```python
from build123d import *

# Parameters (mm, degrees)
BOSS_EXTRUDE1_DEPTH     = 50.8
SKETCH3_R               = 4.9022
CUT_EXTRUDE1_DEPTH      = 50.8
SKETCH4_R               = 1.4732
CUT_EXTRUDE2_DEPTH      = 50.8
FILLET1_R               = 2.54
SKETCH5_W               = 25.4
SKETCH5_H               = 31.75
CUT_EXTRUDE3_DEPTH      = 27.924
CUT_EXTRUDE3_DEPTH_BACK = 5.826


with BuildPart() as part:
    # Sketch2 → Boss-Extrude1 (new body)
    with BuildSketch(Plane(origin=(0, 0, 0), x_dir=(0, 0, -1), z_dir=(1, 0, 0))):
        Polygon((0, 0), (31.75, 0), (31.75, 31.75), (26.924, 31.75), (26.924, 4.826), (0, 4.826), align=None)
    extrude(amount=-BOSS_EXTRUDE1_DEPTH)

    # Sketch3 → Cut-Extrude1 (cut)
    with BuildSketch(Plane.XY.offset(-26.924)):
        with Locations((-38.1, 19.05)):
            Circle(SKETCH3_R)
        with Locations((-12.7, 19.05)):
            Circle(SKETCH3_R)
    extrude(amount=-CUT_EXTRUDE1_DEPTH, mode=Mode.SUBTRACT)

    # Sketch4 → Cut-Extrude2 (cut)
    with BuildSketch(Plane(origin=(0, 4.826, 0), x_dir=(1, 0, 0), z_dir=(0, 1, 0))):
        with Locations((-44.45, 12.7)):
            Circle(SKETCH4_R)
        with Locations((-31.75, 12.7)):
            Circle(SKETCH4_R)
    extrude(amount=-CUT_EXTRUDE2_DEPTH, mode=Mode.SUBTRACT)

    # Fillet1
    fillet1_edges = [part.edges().sort_by_distance(p)[0] for p in [
        (-25.4, 4.826, 0),
        (-25.4, 31.75, -26.924),
    ]]
    fillet(fillet1_edges, radius=FILLET1_R)

    # Sketch5 → Cut-Extrude3 (cut, two sides)
    with BuildSketch(Plane.XY.offset(-26.924)) as cut_extrude3_sk:
        with Locations((-12.7, 15.875)):
            Rectangle(SKETCH5_W, SKETCH5_H)
    extrude(amount=CUT_EXTRUDE3_DEPTH, mode=Mode.SUBTRACT)
    extrude(cut_extrude3_sk.sketch, amount=-CUT_EXTRUDE3_DEPTH_BACK, mode=Mode.SUBTRACT)


solid = part.part
```
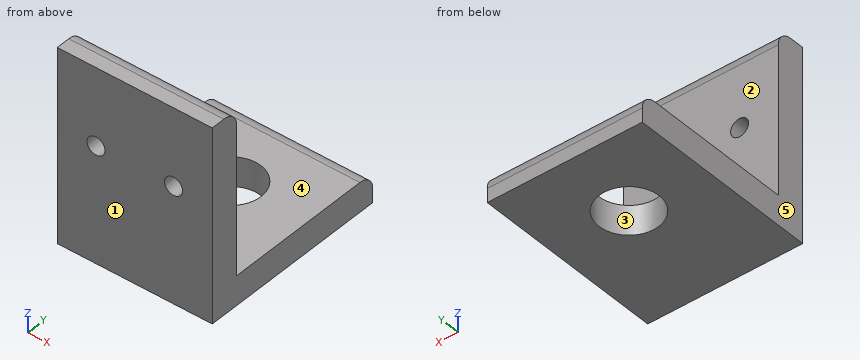
Input: part model. Units: mm. Frame: model coordinates. Face numbers are marked on the shaded views. A direction names the side the tool comes from. Round coordinates to 2 decimals unless told otherwise and drop trailing zeros. Order: outer loops, then holes, each group sorted by start corner. A loop starts at its lowest first (then second) coordinate and runs counter-clockwise, first axis right, second up. Notation, with made-up numbers: (83, 86.5) - (100, 86.5) arc R15 cw to (100, 101.5) - close; hole circle Ø5 at (26.25, 0.5). An arc over 180 degrees is marked (long way). Answer in a Markdown table with one row per item.
Item 1: Section query D-D (x = -48). Return the cut outline in (y, z), then the cut area to 3 significant figures.
Model answer:
| item | result |
|---|---|
| outline | (0, -31.75) - (31.75, -31.75) - (31.75, -29.46) arc R2.54 ccw to (29.21, -26.92) - (4.83, -26.92) - (4.83, -2.54) arc R2.54 ccw to (2.29, 0) - (0, 0) - close |
| area | 280 mm² |
Item 2: Line query: line 1 (X direction, y = 1.4, z = -12.7); line 2 (Z direction, x = -31.75, y = 1.15); line 3 (X direction, y = 1, z = -12). Output: solid intervals per line, ascending.
Model answer:
| item | result |
|---|---|
| line 1 | x = -50.8 to -45.92, -42.98 to -33.22, -30.28 to -25.4 |
| line 2 | z = -31.75 to -14.17, -11.23 to 0 |
| line 3 | x = -50.8 to -45.75, -43.15 to -33.05, -30.45 to -25.4 |
Item 3: Mould query, pull axis X, two halves, no side actions, for the marked faces 3, 4 and 5. Classes: released by +X, released by -X, zero draft, split by the parting line, or undercut.
Model answer:
| item | result |
|---|---|
| face 3 | undercut |
| face 4 | zero draft |
| face 5 | released by -X |
Item 4: Pin query (flat end, axial travel): pin 1 (10 mm diameter, centred on x = -36.5, z = -10, fed in from +Y); pin 2 (12 mm diameter, centred on x = -39.5, y = 22, fed in from +Z); pin 3 (1.8 mm diameter, centred on x = -44.45, z = -12.7, fed in from +Y). Return the tip coordinate at first contact, or that it passes through.
Model answer:
| item | result |
|---|---|
| pin 1 | stops at y = 4.83 |
| pin 2 | stops at z = -26.92 |
| pin 3 | passes through |
Item 5: Section query A-A (z = -12.7). Return the cut outline in (x, y), then the cut area to 3 significant figures.
Model answer:
| item | result |
|---|---|
| outline | (-50.8, 0) - (-45.92, 0) - (-45.92, 4.83) - (-50.8, 4.83) - close; (-42.98, 0) - (-33.22, 0) - (-33.22, 4.83) - (-42.98, 4.83) - close; (-30.28, 0) - (-25.4, 0) - (-25.4, 4.83) - (-30.28, 4.83) - close |
| area | 94.1 mm² |
Item 6: Section query B-B (x = -38.1). Return the cut outline in (y, z), then the cut area to 3 significant figures.
Model answer:
| item | result |
|---|---|
| outline | (0, -31.75) - (14.15, -31.75) - (14.15, -26.92) - (4.83, -26.92) - (4.83, -2.54) arc R2.54 ccw to (2.29, 0) - (0, 0) - close; (23.95, -31.75) - (31.75, -31.75) - (31.75, -29.46) arc R2.54 ccw to (29.21, -26.92) - (23.95, -26.92) - close |
| area | 233 mm² |
Item 7: Section query C-C (y = 19.05). Return the cut outline in (x, z), then the cut area to 3 significant figures.
Model answer:
| item | result |
|---|---|
| outline | (-50.8, -31.75) - (-43, -31.75) - (-43, -26.92) - (-50.8, -26.92) - close; (-33.2, -31.75) - (-25.4, -31.75) - (-25.4, -26.92) - (-33.2, -26.92) - close |
| area | 75.3 mm² |
Item 8: Reachability of the marked faces 1 and 2 from +Z, -Z, +X, -X, +Y, -Y: full face, straight path, thin tool, end or side. Return the list, or none.
Model answer:
| item | result |
|---|---|
| face 1 | +Z, -Z, +X, -X, -Y |
| face 2 | +Z, +X, -X, +Y |
